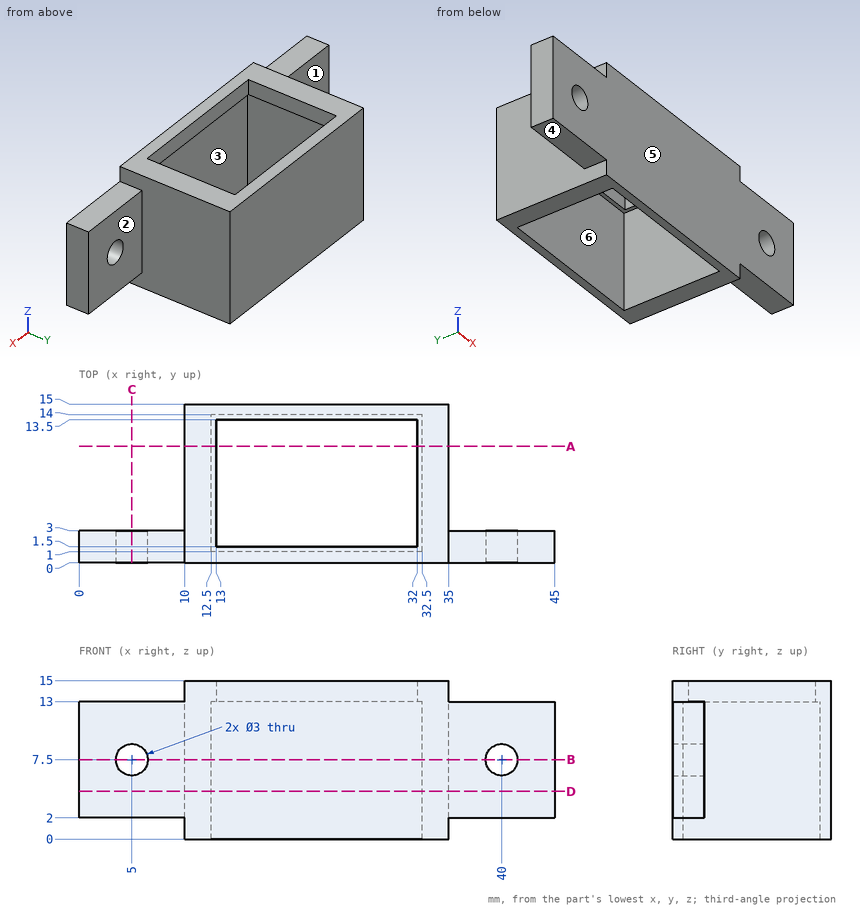
Input: dimensioned drawing with shaded views. Units: mm. Origin: part minimum x, y, z. A direction names the side the tool comes from. Coordinates: 2 decimals unless noted, no trailing zeros. Loops run counter-clockwise (first coordinate to the right, second up) from the corner with the lowest first, then second, coordinate; pieces in that order, holes last. Notation, with made-up numbers: M 15,-9 L 64,-9 A24 ccw 64,9 Z; hole C 3.5,-4.5 d5. An arc over 180 degrees is marked long. One line per item, written item: value. Start each with the question number.
1) Cut plane C-C (x = 5). Return loops of the section in (y, z).
2) Cut plane B-B (z = 7.5). Return loops of the section in (x, y).
3) Draft query along Y for the marked faces 4, 5 and 6. Return one class per face: released by +Y, released by -Y, zero draft, split by the parting line, or undercut.
4) Cut plane A-A (y = 11). Return loops of the section in (x, z).
5) Material intervals for L1, parallel to Z at x = 5, y = 0.6; L2, parallel to Y at x = 17, z = 5.5; L3, parallel to X at y = 7.75, z = 6.5, sorted ascending. Write a range as from..to.
6) Cut plane D-D (z = 4.5). Return loops of the section in (x, y), then the cut area to 3 significant figures.
7) Pin query (flat end, axial travel): P1, Ø1.5, axis at x = 31.5, z = 12.5, coming from the -Y side; P2, Ø1, axis at y = 7, z = 2.5, coming from the -X side; P3, Ø8, axis at x = 42, z = 8.5, coming from the +Y side; P4, Ø0.9, axis at x = 2.5, y = 2, coming from the -Z side. Return the tip coordinate at first contact, or that it passes through.
8) Reachability of the marked faces 1, 2 and 3 from +Z, -Z, +X, -X, +Y, -Y: full face, straight path, thin tool, end or side. Return the list, or none.
Evaluation:
1. outline: M 0,2 L 3,2 L 3,6 L 0,6 Z; M 0,9 L 3,9 L 3,13 L 0,13 Z
2. outline: M 0,0 L 3.5,0 L 3.5,3 L 0,3 Z; M 6.5,0 L 38.5,0 L 38.5,3 L 35,3 L 35,15 L 10,15 L 10,3 L 6.5,3 Z; M 41.5,0 L 45,0 L 45,3 L 41.5,3 Z; hole M 12.5,1 L 32.5,1 L 32.5,14 L 12.5,14 Z
3. face 4: zero draft
3. face 5: released by -Y
3. face 6: undercut
4. outline: M 10,0 L 12.5,0 L 12.5,13 L 13,13 L 13,15 L 10,15 Z; M 32,13 L 32.5,13 L 32.5,0 L 35,0 L 35,15 L 32,15 Z
5. L1: 2..6, 9..13
5. L2: 0..1, 14..15
5. L3: 10..12.5, 32.5..35
6. outline: M 0,0 L 45,0 L 45,3 L 35,3 L 35,15 L 10,15 L 10,3 L 0,3 Z; hole M 12.5,1 L 32.5,1 L 32.5,14 L 12.5,14 Z
6. area: 175 mm^2
7. P1: y = 0
7. P2: x = 10
7. P3: y = 3
7. P4: z = 2
8. face 1: +Z, -Z, -X, +Y
8. face 2: +Z, -Z, +X, +Y
8. face 3: -Z
